The model under review builds one solid part; all positions refer to its coordinate system, in mm. A direction names the side the tool comes from. Round coordinates to 2 decimals unless told otherwise and drop trailing zeros. Order: outer loops, then holes, each group sorted by start corner. A loop starts at its lowest first (then second) coordinate and runs counter-clockwise, first axis right, second up.
from build123d import *

# Parameters (mm, degrees)
IZIM1_R                     = 1.5
Y_KSEKLIK_EKSTR_ZYON1_DEPTH = 5
Y_KSEKLIK_EKSTR_ZYON2_START = -5
IZIM1_2_R                   = 1.5
Y_KSEKLIK_EKSTR_ZYON2_DEPTH = 7


with BuildPart() as part:
    # izim1 → Y_kseklik-Ekstr_zyon1 (new body)
    with BuildSketch(Plane(origin=(0, 0, 0), x_dir=(1, 0, 0), z_dir=(0, 1, 0))):
        Polygon((1.58771324, -2.75), (3.175426481, 0), (1.58771324, 2.75), (-1.58771324, 2.75), (-3.175426481, 0), (-1.58771324, -2.75), align=None)
        with Locations(Location((0, 0, 0), (0, 0, 270))):
            Circle(IZIM1_R, mode=Mode.SUBTRACT)
    extrude(amount=Y_KSEKLIK_EKSTR_ZYON1_DEPTH)

    # izim1_2 → Y_kseklik-Ekstr_zyon2 (add)
    with BuildSketch(Plane(origin=(0, 0, 0), x_dir=(1, 0, 0), z_dir=(0, 1, 0)).offset(Y_KSEKLIK_EKSTR_ZYON2_START)):
        with Locations(Location((0, 0, 0), (0, 0, 270))):
            Circle(IZIM1_2_R)
    extrude(amount=Y_KSEKLIK_EKSTR_ZYON2_DEPTH)


solid = part.part
(1) We need section B-B (x = 0). Give the boundary of the cut face in (y, z).
(2) The part is to be moulded in two halves that separate along Z. For faces 1 (the flat face through (0, 2, 0)), 2 (the flat face through (1.4, 5, -1.3)), 3 (the flat face through (0, 2, -2.75)), say which applies: pulls with the +Z half, pulls with the -Z half, needs draft (parallel to the pull), parting line crosses it, or undercut.
(3) We need section C-C (z = -1.2). Give the boundary of the cut face in (x, y).
(4) To check wall thickness, follow L1, parallel to Y at x = -0.5, z = 1.05; L2, parallel to X at y = 4.25, z = -0.75; L3, parallel to Y at x = 1, z = -1.35. State the ranges of each line that lie inside material, in increasing order.
(5) We need section D-D (y = -2.5). Give the boundary of the cut face in (x, z), and give its area (3 significant figures).
(6) Clearance check with a flat-ended pin moving along its axis: P1, Ø1.5, axis at x = 0.5, z = -0.5, coming from the +Y side. State where the tip first meets the part, or that it passes through.
(7) We need section A-A (y = 3). Give the boundary of the cut face in (x, z), and give its area (3 significant figures).
(8) Tool access review of faces 4 (the flat face through (1.4, 0, -1.3)), 5 (the flat face through (-2.37, 2.465, -1.394)), 6 (the cylindrical face through (0.45, 3.48, 1.43)): name each direction out of +Z, -Z, +X, -X, +Y, -Y from which nothing blocks a thin tool from reaching the whole face with its end or side.
Verdict:
1. outline: (-5, -1.5) - (0, -1.5) - (0, -2.75) - (5, -2.75) - (5, -1.5) - (2, -1.5) - (2, 1.5) - (5, 1.5) - (5, 2.75) - (0, 2.75) - (0, 1.5) - (-5, 1.5) - close
2. face 1: undercut
2. face 2: needs draft
2. face 3: pulls with the -Z half
3. outline: (-2.48, 0) - (-0.9, 0) - (-0.9, -5) - (0.9, -5) - (0.9, 0) - (2.48, 0) - (2.48, 5) - (0.9, 5) - (0.9, 2) - (-0.9, 2) - (-0.9, 5) - (-2.48, 5) - close
4. L1: y = -5 to 2
4. L2: x = -2.74 to -1.3, 1.3 to 2.74
4. L3: y = 0 to 5
5. outline: circle Ø3 at (0, 0)
5. area: 7.07 mm2
6. P1: stops at y = 2
7. outline: (-3.18, 0) - (-1.59, -2.75) - (1.59, -2.75) - (3.18, 0) - (1.59, 2.75) - (-1.59, 2.75) - close; hole circle Ø3 at (0, 0)
7. area: 19.1 mm2
8. face 4: -Y
8. face 5: -Z, -X, +Y, -Y
8. face 6: +Y
